from build123d import *

# Parameters (mm, degrees)
SKETCH1_W           = 70
SKETCH1_H           = 22
BOSS_EXTRUDE1_DEPTH = 10
SKETCH2_R           = 2.25
CUT_EXTRUDE1_DEPTH  = 45
SKETCH3_R           = 3.25
CUT_EXTRUDE2_DEPTH  = 45
SKETCH4_R           = 5.199573864
SKETCH4_R_2         = 3.199573864
SKETCH4_R_3         = 5.25
SKETCH4_R_4         = 3.25
BOSS_EXTRUDE2_DEPTH = 4
SKETCH5_R           = 4
CUT_EXTRUDE3_DEPTH  = 4


with BuildPart() as part:
    # Sketch1 → Boss-Extrude1 (new body)
    with BuildSketch(Plane.XY):
        Rectangle(SKETCH1_W, SKETCH1_H)
    extrude(amount=BOSS_EXTRUDE1_DEPTH)

    # Sketch2 → Cut-Extrude1 (cut)
    with BuildSketch(Plane(origin=(0, 11, 0), x_dir=(1, 0, 0), z_dir=(0, 1, 0))):
        with Locations(Location((-30, -5, 0), (0, 0, 270))):
            Circle(SKETCH2_R)
        with Locations(Location((30, -5, 0), (0, 0, 270))):
            Circle(SKETCH2_R)
    extrude(amount=-CUT_EXTRUDE1_DEPTH, mode=Mode.SUBTRACT)

    # Sketch3 → Cut-Extrude2 (cut)
    with BuildSketch(Plane.XY.offset(10)):
        with Locations((20, 0)):
            Circle(SKETCH3_R)
        with Locations((-20, 0)):
            Circle(SKETCH3_R)
    extrude(amount=-CUT_EXTRUDE2_DEPTH, mode=Mode.SUBTRACT)

    # Sketch4 → Boss-Extrude2 (add)
    # profile 1 of 2: a face of its own
    with BuildSketch(Plane(origin=(0, 0, 0), x_dir=(-1, 0, 0), z_dir=(0, 0, -1))):
        with Locations((-20, 0)):
            Circle(SKETCH4_R)
        with Locations((-20, 0)):
            Circle(SKETCH4_R_2, mode=Mode.SUBTRACT)
    # profile 2 of 2: a face of its own
    with BuildSketch(Plane(origin=(0, 0, 0), x_dir=(-1, 0, 0), z_dir=(0, 0, -1))):
        with Locations((20, 0)):
            Circle(SKETCH4_R_3)
        with Locations(Location((20, 0, 0), (0, 0, 180))):
            Circle(SKETCH4_R_4, mode=Mode.SUBTRACT)
    extrude(amount=BOSS_EXTRUDE2_DEPTH)

    # Sketch5 → Cut-Extrude3 (cut)
    with BuildSketch(Plane.XZ.offset(11)):
        with Locations(Location((30, 5, 0), (0, 0, 270))):
            Circle(SKETCH5_R)
        with Locations(Location((-30, 5, 0), (0, 0, 270))):
            Circle(SKETCH5_R)
    extrude(amount=-CUT_EXTRUDE3_DEPTH, mode=Mode.SUBTRACT)


solid = part.part
Input: part model. Units: mm. Frame: model coordinates. A direction names the side the tool comes from. Give positions to 0.01 mm unless a question says otherwise; leave off trailing zeros. Loops run counter-clockwise (first coordinate to the right, second up) from the corner with the lowest first, then second, coordinate; pieces in that order, holes last. Notation, with made-up numbers: (49, 13.25) -> (97, 13.25) arc R22 ccw to (97, 26.25) -> close; hole circle Ø5 at (-4, 65). An arc over 180 degrees is marked (long way). Answer as a JSON object with one key per item and string values. Group by question number.
Item 1: Cut plane D-D, the plane z = -2. Return the cut outline in (x, y), and give its area (3 significant figures).
Item 2: Cut plane C-C, the plane x = 30. Return the cut outline in (y, z), and give its area (3 significant figures).
Item 3: Line query: probe 1 along X at (y, z) = (10.25, 5); probe 2 along X at (y, z) = (2, 5); probe 3 along X at (y, z) = (-8.5, 1.5). Output: solid intervals per line, ascending.
Item 4: Pin query (flat end, axial travel): P1, Ø2.5, axis at x = 30, z = 5, coming from the +Y side; P2, Ø4, axis at x = -29.5, z = 5, coming from the -Y side; P3, Ø10, axis at x = 8, y = 4, coming from the -Z side. Return the tip coordinate at first contact, or that it passes through.
Item 5: Cut plane A-A, the plane y = 0. Return the cut outline in (x, z), and give its area (3 significant figures).
Item 6: Cut plane B-B, the plane z = 5. Return the cut outline in (x, y), and give its area (3 significant figures).
Item 7: Reachability of faces 4 (the cylindrical face through (-31.996, 2.126, 6.038)), 5 (the cylindrical face through (33.966, -9.028, 5.521)), 6 (the flat face through (20.1, -3.4, -4)), 7 (the cylindrical face through (15.04, 1.56, -1.97)), 8 (the cylindrical face through (16.753, 0.143, 5.07)) from +Z, -Z, +X, -X, +Y, -Y: full face, straight path, thin tool, end or side. Return the list, or none.
Item 8: Pull-direction query (X, two-part tool) for faces 1 (the flat face through (35, 0, 5)), 2 (the flat face through (0, 11, 5)), 3 (the cylindrical face through (23.2, 0.1, -2)); classes: released by +X, released by -X, zero draft, split by the parting line, or undercut.
Checks:
{
 "1": {"outline": "circle Ø10.5 at (-20, 0); circle Ø10.4 at (20, 0); hole circle Ø6.5 at (-20, 0); hole circle Ø6.4 at (20, 0)", "area": "106 mm²"},
 "2": {"outline": "(-11, 0) -> (11, 0) -> (11, 2.75) -> (-7, 2.75) -> (-7, 1) -> (-11, 1) -> close; (-11, 9) -> (-7, 9) -> (-7, 7.25) -> (11, 7.25) -> (11, 10) -> (-11, 10) -> close", "area": "107 mm²"},
 "3": {"probe 1": "x = -35 to -32.25, -27.75 to 27.75, 32.25 to 35", "probe 2": "x = -35 to -32.25, -27.75 to -22.56, -17.44 to 17.44, 22.56 to 27.75, 32.25 to 35", "probe 3": "x = -35 to -31.94, -28.06 to 28.06, 31.94 to 35"},
 "4": {"P1": "passes through", "P2": "stops at y = -7", "P3": "stops at z = 0"},
 "5": {"outline": "(-35, 0) -> (-25.25, 0) -> (-25.25, -4) -> (-23.25, -4) -> (-23.25, 10) -> (-35, 10) -> close; (-16.75, -4) -> (-14.75, -4) -> (-14.75, 0) -> (14.8, 0) -> (14.8, -4) -> (16.8, -4) -> (16.8, 0) -> (16.75, 0) -> (16.75, 10) -> (-16.75, 10) -> close; (23.2, -4) -> (25.2, -4) -> (25.2, 0) -> (35, 0) -> (35, 10) -> (23.25, 10) -> (23.25, 0) -> (23.2, 0) -> close; hole circle Ø4.5 at (-30, 5); hole circle Ø4.5 at (30, 5)", "area": "570 mm²"},
 "6": {"outline": "(-35, -11) -> (-34, -11) -> (-34, -7) -> (-32.25, -7) -> (-32.25, 11) -> (-35, 11) -> close; (-27.75, -7) -> (-26, -7) -> (-26, -11) -> (26, -11) -> (26, -7) -> (27.75, -7) -> (27.75, 11) -> (-27.75, 11) -> close; (32.25, -7) -> (34, -7) -> (34, -11) -> (35, -11) -> (35, 11) -> (32.25, 11) -> close; hole circle Ø6.5 at (-20, 0); hole circle Ø6.5 at (20, 0)", "area": "1,250 mm²"},
 "7": {"face 4": "+Y, -Y", "face 5": "-Y", "face 6": "-Z, +X, -X, +Y, -Y", "face 7": "-Z", "face 8": "+Z"},
 "8": {"face 1": "released by +X", "face 2": "zero draft", "face 3": "undercut"}
}
